```python
from build123d import *

# Parameters (mm, degrees)
F1_DEPTH = 10
F2_DEPTH = 1.8
F3_DEPTH = 5


with BuildPart() as f1:
    # F0 (on Front) → F1 (new body)
    with BuildSketch(Plane.XZ):
        with BuildLine():
            Line((-5, -2.5), (-5, 2.5))
            ThreePointArc((-5, 2.5), (-5.968249, 3.331751), (-6.8, 4.3))
            Line((-6.8, 4.3), (-6.8, -4.3))
            Line((-6.8, -4.3), (6.8, -4.3))
            Line((6.8, -4.3), (6.8, 4.3))
            ThreePointArc((6.8, 4.3), (5.968249, 3.331751), (5, 2.5))
            Line((5, 2.5), (5, -2.5))
            Line((5, -2.5), (-5, -2.5))
        make_face()
        with BuildLine():
            ThreePointArc((-6.8, 4.3), (-5.968249, 3.331751), (-5, 2.5))
            Line((-5, 2.5), (5, 2.5))
            ThreePointArc((5, 2.5), (5.968249, 3.331751), (6.8, 4.3))
            Line((6.8, 4.3), (0, 4.3))
            Line((0, 4.3), (-6.8, 4.3))
        make_face()
    extrude(amount=F1_DEPTH)

    # F0 (on Front) → F2 (join)
    with BuildSketch(Plane.XZ):
        with BuildLine():
            Line((5, 2.5), (-5, 2.5))
            ThreePointArc((-5, 2.5), (0, 0.859621), (5, 2.5))
        make_face()
        with BuildLine():
            ThreePointArc((5, 2.5), (0, 0.859621), (-5, 2.5))
            Line((-5, 2.5), (-5, -2.5))
            Line((-5, -2.5), (5, -2.5))
            Line((5, -2.5), (5, 2.5))
        make_face()
    extrude(amount=F2_DEPTH)

    # F0 (on Front) → F3 (join)
    with BuildSketch(Plane.XZ):
        with BuildLine():
            Line((0, 4.3), (6.8, 4.3))
            ThreePointArc((6.8, 4.3), (2.631105, 17.319806), (-8.440379, 9.3))
            Line((-8.440379, 9.3), (-5, 9.3))
            ThreePointArc((-5, 9.3), (3.535534, 12.835534), (0, 4.3))
        make_face()
    extrude(amount=F3_DEPTH)


solid = f1.part
```
Verification items for the finished model (mm, model axes). A direction names the side the tool comes from. Give positions to 0.01 mm unless a question says otherwise; leave off trailing zeros. Loops run counter-clockwise (first coordinate to the right, second up) from the corner with the lowest first, then second, coordinate; pieces in that order, holes last.
1. Mould release check, pull along Z, two halves, no side actions. Record for faces 1 (the cylindrical face through (2.84, -2.46, 17.25)), 2 (the flat face through (-7, -2, 9.3)), 3 (the flat face through (4, -5, 14)): released by +Z, released by -Z, zero draft, split by the parting line, or undercut.
2. Go/stop test with flat-tipped pins: pin 1 Ø2.5 at (y, z) = (-5.5, -0.5) entering from +X; pin 2 Ø3 at (x, y) = (-2, -3.5) entering from +Z; pin 3 Ø2 at (x, y) = (4.5, -4.5) entering from +Z. Record where each tip stops, or that it passes through.
3. Section check D-D, the plane z = -1.75. Enter the section's corners in (x, y), then the cut area to 3 significant figures.
4. Section check C-C, the plane x = -1.75. Enter the section's corners in (y, z), then the cut area to 3 significant figures.
5. Section check B-B, the plane z = 10.5. Enter the section's corners in (x, y).
6. Thickness scan on line 1 (Z direction, x = -2, y = -5.5); line 2 (Z direction, x = -3.75, y = -3.75); line 3 (X direction, y = -5, z = 1.5). Record the ranges inside material, lowest first.
7. Set-up check for faces 4 (the flat face through (6.8, -5, 0)), 5 (the flat face through (0, -6, -2.5)), 6 (the flat face through (2, 0, 4)), 7 (the flat face through (-6.8, -5, 0)), 8 (the flat face through (-1, -6, 4.3)): record each of +Z, -Z, +X, -X, +Y, -Y from which the full face is reachable in a straight line by a thin tool's end or side.
8. Section check A-A, the plane y = -7.25. Enter the section's corners in (x, z), then the cut area to 3 significant figures.
Geometry says:
1. face 1: split by the parting line
1. face 2: undercut
1. face 3: zero draft
2. pin 1: stops at x = 6.8
2. pin 2: stops at z = 17.73
2. pin 3: stops at z = 16.98
3. outline: (-6.8, -10) - (-5, -10) - (-5, -1.8) - (5, -1.8) - (5, -10) - (6.8, -10) - (6.8, 0) - (-6.8, 0) - close
3. area: 54.0 mm2
4. outline: (-10, -4.3) - (0, -4.3) - (0, 4.3) - (-10, 4.3) - (-10, 2.5) - (-1.8, 2.5) - (-1.8, -2.5) - (-10, -2.5) - close; (-5, 13.98) - (0, 13.98) - (0, 17.56) - (-5, 17.56) - close
4. area: 62.9 mm2
5. outline: (-8.35, -5) - (-4.85, -5) - (-4.85, 0) - (-8.35, 0) - close; (4.85, -5) - (8.35, -5) - (8.35, 0) - (4.85, 0) - close
6. line 1: z = -4.3 to -2.5, 2.5 to 4.3
6. line 2: z = -4.3 to -2.5, 2.5 to 4.3, 12.61 to 16.86
6. line 3: x = -6.8 to -5, 5 to 6.8
7. face 4: -Z, +X, +Y, -Y
7. face 5: -Y
7. face 6: +Z, -Z, +X, -X, +Y
7. face 7: -Z, -X, +Y, -Y
7. face 8: -X, -Y
8. outline: (-6.8, -4.3) - (6.8, -4.3) - (6.8, 4.3) - (-6.8, 4.3) - close; hole (-5, -2.5) - (5, -2.5) - (5, 2.5) - (-5, 2.5) - close
8. area: 67.0 mm2
